Autodesk Inventor part; units mm, degrees
ref_plane "Arbeitsebene2" through (-9.2536, 3.4368, 4) normal (0, 0, 1) x (1, -0.0003, 0)
ref_plane "YZ Plane" through (0, 0, 0) normal (1, 0, 0) x (0, 1, 0)
ref_plane "XZ Plane" through (0, 0, 0) normal (0, 1, 0) x (-1, 0, 0)
ref_plane "Arbeitsebene1" through (0, 0, 0) normal (0, 0, 1) x (1, 0, 0)
sketch "Skizze1" plane through (0, 0, 0) normal (0, 0, 1) x (1, 0, 0)
  line L0 (-7.7466, -5.9177) -> (-1.7466, -5.9177)
  line L1 (-1.7466, -5.9177) -> (-1.7466, 2.0823)
  line L2 (-1.7466, 2.0823) -> (-7.7466, 2.0823)
  line L3 (-7.7466, 2.0823) -> (-7.7466, -5.9177)
  line L4 (-7.7466, -5.9177) -> (-1.7466, 2.0823) construction
  line L5 (-1.7466, -5.9177) -> (-7.7466, 2.0823) construction
  line L6 (-7.7466, -5.9177) -> (-1.7466, -5.9177)
  line L7 (-1.7466, -5.9177) -> (-1.7466, -3.9177)
  line L8 (-1.7466, -3.9177) -> (-7.7466, -3.9177)
  line L9 (-7.7466, -3.9177) -> (-7.7466, -5.9177)
  circle A0 centre (-4.7466, -1.9177) radius 1.6
  line L10 (0.5034, 22.0823) -> (-10.1632, 22.0823)
  line L11 (-10.1632, 22.0823) -> (-10.1632, 2.0823)
  line L12 (-10.1632, 2.0823) -> (0.5034, 2.0823)
  line L13 (0.5034, 2.0823) -> (0.5034, 22.0823)
  line L14 (0.5034, 22.0823) -> (-10.1632, 2.0823) construction
  line L15 (-10.1632, 22.0823) -> (0.5034, 2.0823) construction
  circle A1 centre (-4.7466, 17.0823) radius 1.6
  circle A2 centre (-4.4966, 8.0823) radius 4.1
  line L16 (-7.7466, -5.9177) -> (-10.1632, -5.9177)
  line L17 (-10.1632, -5.9177) -> (-10.1632, 2.0823)
  line L18 (-10.1632, 2.0823) -> (-7.7466, 2.0823)
  line L19 (-7.7466, 2.0823) -> (-7.7466, -5.9177)
  line L20 (-10.1632, -5.9177) -> (-12.7262, -5.9177)
  line L21 (-12.7262, -5.9177) -> (-12.7262, 22.0823)
  line L22 (-12.7262, 22.0823) -> (-10.1632, 22.0823)
  line L23 (-10.1632, 22.0823) -> (-10.1632, -5.9177)
  point P0 (0, 0)
  point P1 (-7.7466, -3.9177)
  point P2 (-4.8299, 12.0823)
  point P3 (-1.7466, 2.0823)
  point P4 (-7.7466, 2.0823)
  point P5 (-4.7466, 2.0823)
  dimension "d0" = 6
  dimension "d1" = 8
  dimension "d10" = 2
  dimension "d11" = 3.2
  dimension "d12" = 20
  dimension "d13" = 3.2
  dimension "d14" = 19
  dimension "d15" = 8.2
  dimension "d44" = 0
  dimension "d45" = 5.25
  dimension "d46" = 9
  dimension "d53" = 0.25
ref_plane "Arbeitsebene2" through (-9.2536, 3.4368, 4) normal (0, 0, 1) x (1, -0.0003, 0)
extrude "Extrusion1" add sketch "Skizze1" along normal blind 1.5 contours L16 L17 L12 L3 | L3 L2 L1 L8 | L20 L21 L22 L11 L17 | L12 L11 L10 L13 L2
sketch "Skizze4" plane through (0, 0, 1.5) normal (0, 0, 1) x (1, 0, 0)
  line L0 (-55.6662, 35.6355) -> (-7.4062, 35.6355) construction
  line L1 (-7.4062, 35.6355) -> (-7.4062, -28.7112) construction
  line L2 (-7.4062, -28.7112) -> (-55.6662, -28.7112) construction
  line L3 (-55.6662, -28.7112) -> (-55.6662, 35.6355) construction
  line L4 (-34.8105, 18.9517) -> (-34.8105, 11.3513)
  line L5 (-34.8105, 11.3513) -> (-29.4903, 14.6086)
  line L6 (-1.7466, -3.9177) -> (-1.7466, 2.0823)
  line L7 (-1.7466, 2.0823) -> (0.5034, 2.0823)
  line L8 (0.5034, 2.0823) -> (0.5034, 22.0823)
  line L9 (-7.7466, -5.9177) -> (-7.7466, -3.9177)
  line L10 (-7.7466, -3.9177) -> (-1.7466, -3.9177)
  circle A0 centre (-4.7466, 17.0823) radius 1.6
  circle A1 centre (-4.4966, 8.0823) radius 4.1
  circle A2 centre (-4.7466, -1.9177) radius 1.6
  line L11 (1.3127, 5.8523) -> (-2.2666, 13.8915)
  line L12 (-2.2666, 13.8915) -> (-10.3058, 10.3122)
  line L13 (-10.3058, 10.3122) -> (-6.7265, 2.273)
  line L14 (-6.7265, 2.273) -> (1.3127, 5.8523)
  line L15 (1.3127, 5.8523) -> (-10.3058, 10.3122) construction
  line L16 (-2.2666, 13.8915) -> (-6.7265, 2.273) construction
  line L17 (1.3127, 5.8523) -> (10.1127, 5.8523) construction
  line L18 (0.5034, 22.0823) -> (-12.7262, 22.0823)
  line L19 (-12.7262, 22.0823) -> (-12.7262, -5.9177)
  line L20 (-12.7262, -5.9177) -> (-7.7466, -5.9177)
  line L21 (-7.7466, -3.9177) -> (-1.7466, -3.9177)
  line L22 (-7.7466, -3.9177) -> (-12.7262, -3.9177)
  line L23 (-12.7262, 22.0823) -> (-12.7262, -5.9177)
  point P0 (0, 0)
  point P1 (0.5034, 5.492)
  point P2 (0.5034, 7.6699)
  dimension "d40" = 8.8
  dimension "d41" = 114
  dimension "d42" = 8.8
extrude "Extrusion4" add sketch "Skizze4" along normal blind 2 contours L10 L22 L19 L18 L8 L11 L12 L13 L14 L7 L6
chamfer "Fase2" distance 2 angle 45 1 edges at (-1.7466, 2.0823, 1.75)
properties part number "30_Linear_Stage_NEMA11_baseholder_bayonetmount_objective_autofocus_kes400_camerabracket_underAnAngle"
Verification items for the finished model (mm, model axes). A direction names the side the tool comes from. Give positions to 0.01 mm unless a question says otherwise; leave off trailing zeros. Write each loop counter-clockwise with the first axis right and the second up, starting at its lowest first coordinate (ties: lowest second). Pieces come first, ordered by that corner, then holes. Notation, with made-up numbers: M 69,74 L 85,74 A14 ccw 85,86 Z; hole C 57.5,49.25 d4. An arc over 180 degrees is marked long. Put each result on its own line as item: value. Start each with the question number.
1. Section check B-B (y = -1.25). Record the cut outline in (x, z), and give its area (3 significant figures).
2. Scan lines: line 1 along Y through (x, z) = (-5.75, 0.4); line 2 along Y through (x, z) = (-6, 3.05); line 3 along X through (y, z) = (-0.25, 0.5). Record each from-to range of solid material in increasing order. Write a range as [from, to].
3. Section check A-A (x = -8.25). Record the cut outline in (y, z), and give its area (3 significant figures).
4. Section check D-D (x = -4). Record the cut outline in (y, z).
5. Draft check along X on faces 1 (the face through (-12.726, 8, 2)), 2 (the face through (-8.54, 6.35, 2.49)), 3 (the face through (-8, 12, 3.5)). Enter one of: +X half, -X half, draft (parallel to the pull), parting line (faces both ways), or undercut.
6. Section check C-C (z = 2.85). Record the cut outline in (x, y).
7. Go/stop test with flat-tipped pins: pin 1 Ø2 at (x, y) = (-9.5, -5) entering from +Z; pin 2 Ø1.8 at (y, z) = (-2, 2.5) entering from +X. Record where each tip stops, or that it passes through.
8. Set-up check for faces 4 (the face through (-6, 22.082, 2)), 5 (the face through (-6, 4, 1.5)), 6 (the face through (-10, -5, 1.5)), 7 (the face through (-4.955, 15.496, 1.726)), 8 (the face through (-1.747, -2, 2)): record each of +Z, -Z, +X, -X, +Y, -Y from which the full face is reachable in a straight line by a thin tool's end or side.
Answer list:
1. outline: M -12.73,0 L -6.2,0 L -6.2,3.5 L -12.73,3.5 Z; M -3.29,0 L -1.75,0 L -1.75,3.5 L -3.29,3.5 Z
1. area: 28.3 mm2
2. line 1: [-3.92, -3.16], [-0.67, 4.18], [11.99, 15.84], [18.33, 22.08]
2. line 2: [-3.92, -2.91], [-0.92, 2.6], [12.23, 16.09], [18.08, 22.08]
2. line 3: [-12.73, -1.75]
3. outline: M -5.92,0 L 6.43,0 L 6.43,1.5 L 5.69,1.5 L 5.69,3.5 L -3.92,3.5 L -3.92,1.5 L -5.92,1.5 Z; M 9.73,0 L 22.08,0 L 22.08,3.5 L 11.23,3.5 L 11.23,1.5 L 9.73,1.5 Z
3. area: 78.0 mm2
4. outline: M -3.92,0 L -3.33,0 L -3.33,3.5 L -3.92,3.5 Z; M -0.5,0 L 4.01,0 L 4.01,1.5 L 3.49,1.5 L 3.49,3.5 L -0.5,3.5 Z; M 12.15,0 L 15.67,0 L 15.67,3.5 L 13.12,3.5 L 13.12,1.5 L 12.15,1.5 Z; M 18.5,0 L 22.08,0 L 22.08,3.5 L 18.5,3.5 Z
5. face 1: -X half
5. face 2: undercut
5. face 3: draft
6. outline: M -12.73,-3.92 L -1.75,-3.92 L -1.75,0.08 L 0.25,2.08 L 0.5,2.08 L 0.5,5.49 L -6.73,2.27 L -10.31,10.31 L -2.27,13.89 L 0.5,7.67 L 0.5,22.08 L -12.73,22.08 Z; hole C -4.75,-1.92 d3.2; hole C -4.75,17.08 d3.2
7. pin 1: z = 1.5
7. pin 2: x = -1.75
8. face 4: +Z, -Z, +X, -X, +Y
8. face 5: +Z
8. face 6: +Z, +X, -X, -Y
8. face 7: +Z, -Z
8. face 8: +Z, -Z, +X, -Y
